from build123d import *

# Parameters (mm, degrees)
SKETCH1_W = 2
SKETCH1_H = 1


with BuildPart() as part:
    # Sketch1 → Revolve2 (revolve)
    with BuildSketch(Plane.XY, mode=Mode.PRIVATE) as revolve2_sk:
        with Locations((-1, -0.5)):
            Rectangle(SKETCH1_W, SKETCH1_H)
        Polygon((0, 0), (0, 7), (-3, 7), (-3, 0), (-2, 0), align=None)
        Polygon((0, 7), (0, 9), (-5, 9), (-5, 7), (-3, 7), align=None)
        with BuildLine():
            Line((0, 9), (0, 9.68337521))
            Line((0, 9.68337521), (-1, 9.68337521))
            Line((-1, 9.68337521), (-1, 11.599454993))
            ThreePointArc((-1, 11.599454993), (-3.269448205, 10.714350109), (-5, 9))
            Line((-5, 9), (0, 9))
        make_face()
    revolve(revolve2_sk.sketch.rotate(Axis((0, 85.082557183, 0), (0, -1, 0)), 270), axis=Axis((0, 85.082557183, 0), (0, -1, 0)))


solid = part.part
Design review of the part built by this model. Coordinates are the model's own, in mm. A direction names the side the tool comes from. Coordinates: 2 decimals unless noted, no trailing zeros. Write each loop counter-clockwise with the first axis right and the second up, starting at its lowest first coordinate (ties: lowest second). Pieces come first, ordered by that corner, then holes. Notation, with made-up numbers: (39, 67.25) - (70, 67.25) arc R13 ccw to (70, 91.25) - close; hole circle Ø1 at (-9.75, 35.5). An arc over 180 degrees is marked (long way). Use one line per item in the form item = value.
Q1. Consider section B-B (z = 0). Write out the cut boundary in (x, y), plus the area to 3 significant figures.
Taken from the geometry:
outline = (-5, 7) - (-3, 7) - (-3, 0) - (-2, 0) - (-2, -1) - (2, -1) - (2, 0) - (3, 0) - (3, 7) - (5, 7) - (5, 9) arc R6 ccw to (1, 11.6) - (1, 9.68) - (-1, 9.68) - (-1, 11.6) arc R6 ccw to (-5, 9) - close
area = 80.9 mm^2
Q2. Insertion check: pin 1 Ø1.5 at (x, z) = (-2.5, 1) entering from +Y; pin 2 Ø5 at (x, y) = (-3.5, 9.5) entering from -Z; pin 3 Ø5 at (x, z) = (1, -2.5) entering from -Y; pin 4 Ø1.5 at (x, z) = (1, -2) entering from +Y. Each pin has a flat end and moves straight along its axis. Give the tip position at first contact, or say it passes through.
Taken from the geometry:
pin_1 = 11.36
pin_2 = -4.89
pin_3 = -1
pin_4 = 11.5
Q3. For probe 1 along Y at (x, z) = (-0.5, -0.25); probe 2 along Y at (x, z) = (2.75, -3.5); probe 3 along X at (y, z) = (6.5, -2.5), list the stretches that pass through material, from the lowest coordinate up.
Taken from the geometry:
probe_1 = -1 to 9.68
probe_2 = 7 to 9.71
probe_3 = -1.66 to 1.66
Q4. Consider section D-D (z = 4). Write out the cut boundary in (x, y), plus the area to 3 significant figures.
Taken from the geometry:
outline = (-3, 7) - (3, 7) - (3, 9) arc R4.47 ccw to (-3, 9) - close
area = 16.8 mm^2
Q5. The part is to be moulded in two halves that separate along X. For faces 1 (the cylindrical face through (1, 11, 0)), 2 (the cylindrical face through (4.88, 7.99, -1.08)), 3 (the flat face through (3.3, 7, -0.1)), say which applies: +X half, -X half, draft (parallel to the pull), parting line (faces both ways), or undercut.
Taken from the geometry:
face_1 = undercut
face_2 = parting line
face_3 = draft
Q6. Machinability: for faces 4 (the flat face through (0, 9.683, 0)), 5 (the flat face through (2, 0, 1)), 6 (the flat face through (0, -1, 0)), which of the approach directions +Z, -Z, +X, -X, +Y, -Y give a long, thin tool a straight path to every point of the face, cutting with its end or side? Answer none if there is none.
Taken from the geometry:
face_4 = +Y
face_5 = -Y
face_6 = +Z, -Z, +X, -X, -Y
Q7. Consider section A-A (x = 0). Write out the cut boundary in (y, z).
Taken from the geometry:
outline = (-1, -2) - (0, -2) - (0, -3) - (7, -3) - (7, -5) - (9, -5) arc R6 ccw to (11.6, -1) - (9.68, -1) - (9.68, 1) - (11.6, 1) arc R6 ccw to (9, 5) - (7, 5) - (7, 3) - (0, 3) - (0, 2) - (-1, 2) - close
Q8. Consider section C-C (y = 6.5). Write out the cut boundary in (x, z), plus the area to 3 significant figures.
Taken from the geometry:
outline = circle Ø6 at (0, 0)
area = 28.3 mm^2
